Geometry: see drawing. Coordinates: mm, zero at the bounding-box minimum. A direction names the side the tool comes from. Round coordinates to 2 decimals unless told otherwise and drop trailing zeros. Write each loop counter-clockwise with the first axis right and the second up, starting at its lowest first coordinate (ties: lowest second). Pieces come first, ordered by that corner, then holes. Notation, with made-up numbers: M 3.25,-32.5 L 56.25,-32.5 A27 ccw 56.25,-0.5 Z; hole C 74.5,-30 d10. An arc over 180 degrees is marked long. Use a Markdown table: item, result.
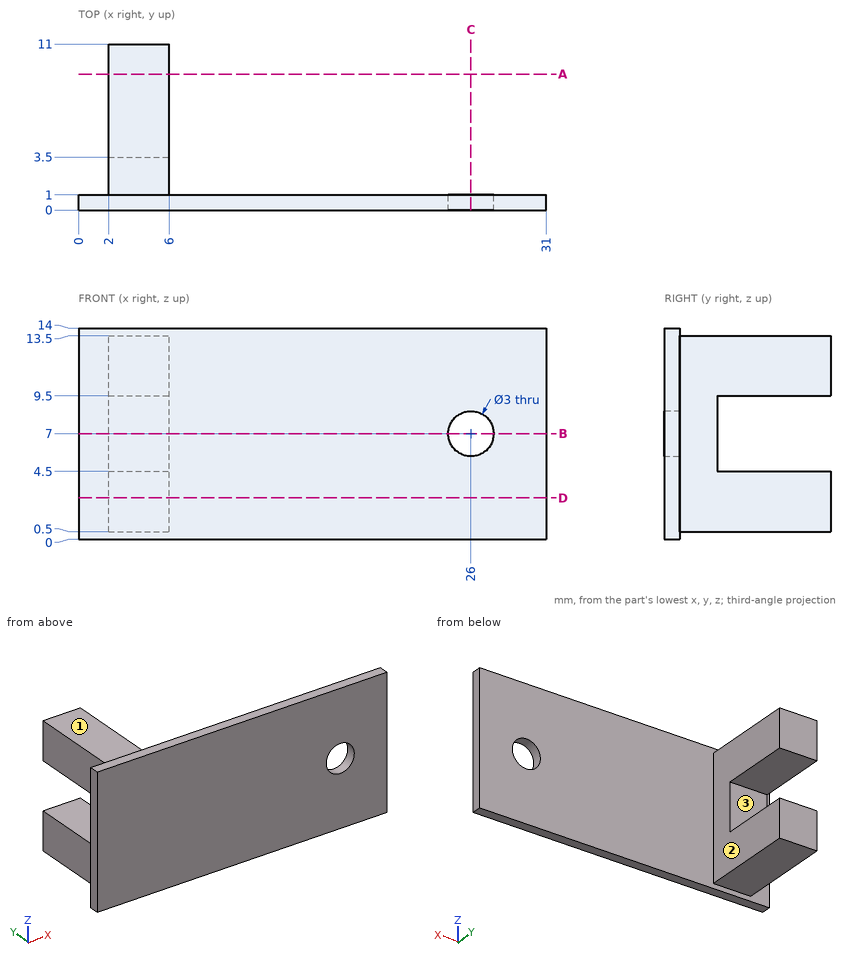
Q1. Section B-B on z = 7. Return loops of the section in (x, y), plus the area to 3 significant figures.
Results are:
| item | result |
|---|---|
| outline | M 0,0 L 24.5,0 L 24.5,1 L 6,1 L 6,3.5 L 2,3.5 L 2,1 L 0,1 Z; M 27.5,0 L 31,0 L 31,1 L 27.5,1 Z |
| area | 38.0 mm^2 |
Q2. Section C-C on x = 26. Return loops of the section in (y, z), plus the area to 3 significant figures.
Results are:
| item | result |
|---|---|
| outline | M 0,0 L 1,0 L 1,5.5 L 0,5.5 Z; M 0,8.5 L 1,8.5 L 1,14 L 0,14 Z |
| area | 11.0 mm^2 |
Q3. Section A-A on y = 9. Return loops of the section in (x, z), plus the area to 3 significant figures.
Results are:
| item | result |
|---|---|
| outline | M 2,0.5 L 6,0.5 L 6,4.5 L 2,4.5 Z; M 2,9.5 L 6,9.5 L 6,13.5 L 2,13.5 Z |
| area | 32.0 mm^2 |
Q4. First-contact query: pin 1 Ø2 at (y, z) = (9, 10.5) entering from -X; pin 2 Ø4 at (x, z) = (19, 4) entering from +Y; pin 3 Ø3 at (x, z) = (6.5, 5.5) entering from -Y; pin 4 Ø3 at (x, y) = (4, 5) entering from -Z. Flat tips, straight axial feed; report the tip coordinate or a pass-through.
Results are:
| item | result |
|---|---|
| pin 1 | x = 2 |
| pin 2 | y = 1 |
| pin 3 | y = 0 |
| pin 4 | z = 0.5 |
Q5. Line query: L1, parallel to X at y = 0.7, z = 7; L2, parallel to Y at x = 14, z = 4.5; L3, parallel to X at y = 8.5, z = 12.75. Output: solid intervals per line, ascending.
Results are:
| item | result |
|---|---|
| L1 | 0 to 24.5, 27.5 to 31 |
| L2 | 0 to 1 |
| L3 | 2 to 6 |
Q6. Reachability of the marked faces 1, 2 and 3 from +Z, -Z, +X, -X, +Y, -Y: full face, straight path, thin tool, end or side. Return the list, or none.
Results are:
| item | result |
|---|---|
| face 1 | +Z, +X, -X, +Y |
| face 2 | +Z, -Z, +X, +Y |
| face 3 | +X, -X, +Y |
Q7. Section D-D on z = 2.75. Return loops of the section in (x, y), plus the area to 3 significant figures.
Results are:
| item | result |
|---|---|
| outline | M 0,0 L 31,0 L 31,1 L 6,1 L 6,11 L 2,11 L 2,1 L 0,1 Z |
| area | 71.0 mm^2 |
